Autodesk Inventor part; units mm, degrees
ref_plane "YZ Plane" through (0, 0, 0) normal (1, 0, 0) x (0, 1, 0)
ref_plane "XZ Plane" through (0, 0, 0) normal (0, 1, 0) x (-1, 0, 0)
ref_plane "XY Plane" through (0, 0, 0) normal (0, 0, 1) x (1, 0, 0)
sketch "Sketch1" plane through (0, 0, 0) normal (0, 0, 1) x (1, 0, 0)
  line L0 (0, 0) -> (19.05, 0)
  line L1 (19.05, 0) -> (19.05, 19.05)
  line L2 (19.05, 19.05) -> (0, 19.05)
  line L3 (0, 19.05) -> (0, 0)
  line L4 (17.4625, 17.4625) -> (1.5875, 17.4625)
  line L5 (1.5875, 17.4625) -> (1.5875, 1.5875)
  line L6 (1.5875, 1.5875) -> (17.4625, 1.5875)
  line L7 (17.4625, 1.5875) -> (17.4625, 17.4625)
  dimension "d0" = 19.05
  dimension "d1" = 19.05
  dimension "d2" = 1.5875
  dimension "d3" = 1.5875
  dimension "d4" = 1.5875
  dimension "d5" = 1.5875
extrude "Extrusion1" add sketch "Sketch1" along normal blind 742.95
sketch "Sketch2" plane through (0, 19.05, 0) normal (0, 1, 0) x (1, 0, 0)
  line L0 (19.05, 0) -> (0, 0)
  line L1 (0, 0) -> (0, -742.95)
  line L2 (19.05, -742.95) -> (0, -742.95)
  line L3 (19.05, -742.95) -> (0, -723.9)
  line L4 (19.05, 0) -> (0, -19.05)
  dimension "d8" = 45
  dimension "d9" = 45
extrude "Extrusion2" cut sketch "Sketch2" against normal through all
equation "\"d3\" = d2"
equation "\"d4\" = d2"
equation "\"d5\" = d3"
properties part number "Bumper Rail Side"
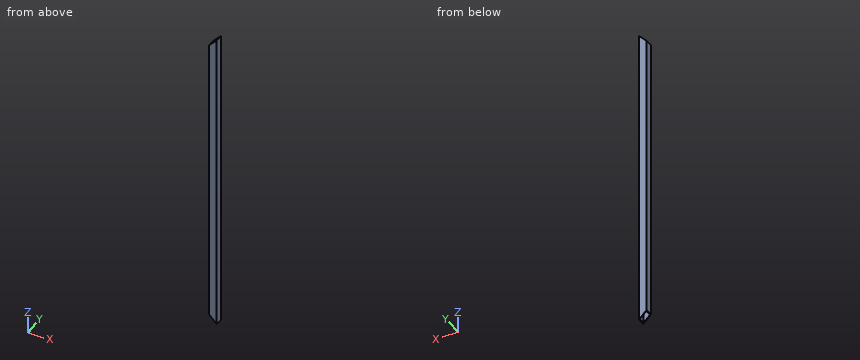
The listing builds one solid part. Answer for the finished solid, in the listing's coordinates (mm). Round coordinates to 2 decimals unless told otherwise and drop trailing zeros. Write each loop counter-clockwise with the first axis right and the second up, starting at its lowest first coordinate (ties: lowest second). Pieces come first, ordered by that corner, then holes. Notation, with made-up numbers: (57, 67.5) - (96, 67.5) arc R15 cw to (96, 81.5) - close; hole circle Ø9 at (2.5, 13.5). An arc over 180 degrees is marked (long way). Use a Markdown table: item, result. Add a question column.
1. The part is cut by section A-A (x = 14.5). Write down the section's boundary in (y, z).
2. Consider line 1 (X direction, y = 13.75, z = 406.5); line 2 (Z direction, x = 5, y = 1.5). Determine where each line is inside the solid, lowest interval first.
3. The part is cut by section C-C (z = 263). Write down the section's boundary in (x, y).
4. The part is cut by section B-B (y = 4.75). Write down the section's boundary in (x, z), and give its area (3 significant figures).
5. Flat-ended cylindrical pins translate along their axes: P1, Ø4, axis at x = 9, y = 3, coming from the +Z side; P2, Ø10, axis at x = 2.5, y = 5, coming from the +Z side; P3, Ø1, axis at x = 9.5, y = 15.5, coming from the +Z side. Find the tip coordinate at first contact, or state that the pin passes through.
Reported:
| question | item | result |
|---|---|---|
| 1 | outline | (0, 4.55) - (1.59, 4.55) - (1.59, 738.4) - (0, 738.4) - close; (17.46, 4.55) - (19.05, 4.55) - (19.05, 738.4) - (17.46, 738.4) - close |
| 2 | line 1 | 0 to 1.59, 17.46 to 19.05 |
| 2 | line 2 | 14.05 to 728.9 |
| 3 | outline | (0, 0) - (19.05, 0) - (19.05, 19.05) - (0, 19.05) - close; hole (1.59, 1.59) - (17.46, 1.59) - (17.46, 17.46) - (1.59, 17.46) - close |
| 4 | outline | (0, 19.05) - (1.59, 17.46) - (1.59, 725.49) - (0, 723.9) - close; (17.46, 1.59) - (19.05, 0) - (19.05, 742.95) - (17.46, 741.36) - close |
| 4 | area | 2,300 mm^2 |
| 5 | P1 | z = 734.32 |
| 5 | P2 | z = 730.05 |
| 5 | P3 | through |
